Geometry check sheet. Reference: the model listing, model coordinates, mm. Face numbers are marked on the shaded views. A direction names the side the tool comes from. Round coordinates to 2 decimals unless told otherwise and drop trailing zeros. Write each loop counter-clockwise with the first axis right and the second up, starting at its lowest first coordinate (ties: lowest second). Pieces come first, ordered by that corner, then holes.
Item 1: Depth check by flat-ended pin: P1, Ø4, axis at x = -7.5, z = -12.5, coming from the +Y side; P2, Ø2, axis at x = 9, y = -10, coming from the -Z side; P3, Ø2, axis at x = -3, y = -20, coming from the +Z side. Enter the tip coordinate at first touch or a pass-through.
Item 2: Cross-section at B-B (y = -6). Enter the section's corners in (x, z), then the cut area to 3 significant figures.
Item 3: Cross-section at C-C (z = 9). Enter the section's corners in (x, y), then the cut area to 3 significant figures.
Item 4: Access from +Z, -Z, +X, -X, +Y, -Y to the whole of each face (thin tool, end or side, straight path). Record for the marked faces 1 and 2.
Item 5: Cross-section at D-D (x = -12.5). Enter the section's corners in (y, z).
Item 6: Scan lines: probe 1 along Y at (x, z) = (0.5, -20); probe 2 along Z at (x, y) = (0, 4); probe 3 along Z at (x, y) = (0.5, -20.5). Record each from-to range of solid material in increasing order.
Item 7: Cross-section at A-A (x = 0). Enter the section's corners in (y, z).
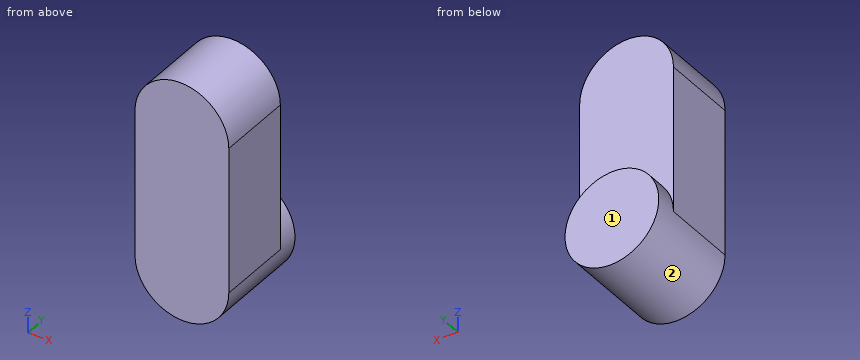
from build123d import *

# Parameters (mm, degrees)
F1_DEPTH = 7.24
F2_DEPTH = 25.4


with BuildPart() as f1:
    # F0 (on Front) → F1 (new body)
    with BuildSketch(Plane.XZ):
        with BuildLine():
            ThreePointArc((-16, -49.9569810927), (0, -65.9569810927), (16, -49.9569810927))
            ThreePointArc((16, -49.9569810927), (0, -33.9569810927), (-16, -49.9569810927))
        make_face()
    extrude(amount=-F1_DEPTH)

    # F0 (on Front) → F2 (join)
    with BuildSketch(Plane.XZ):
        with BuildLine():
            ThreePointArc((-16, 0), (0, -16), (16, 0))
            ThreePointArc((16, 0), (0, 16), (-16, 0))
        make_face()
        with BuildLine():
            Line((16, -49.9569810927), (16, 0))
            ThreePointArc((16, 0), (0, -16), (-16, 0))
            Line((-16, 0), (-16, -49.9569810927))
            ThreePointArc((-16, -49.9569810927), (0, -33.9569810927), (16, -49.9569810927))
        make_face()
        with BuildLine():
            ThreePointArc((-16, -49.9569810927), (0, -65.9569810927), (16, -49.9569810927))
            ThreePointArc((16, -49.9569810927), (0, -33.9569810927), (-16, -49.9569810927))
        make_face()
    extrude(amount=F2_DEPTH)


solid = f1.part
Resolved:
1. P1: stops at y = 0
1. P2: stops at z = -63.81
1. P3: stops at z = 15.87
2. outline: (-16, -49.96) arc R16 ccw to (16, -49.96) - (16, 0) arc R16 ccw to (-16, 0) - close
2. area: 2,400 mm2
3. outline: (-13.23, -25.4) - (13.23, -25.4) - (13.23, 0) - (-13.23, 0) - close
3. area: 672 mm2
4. face 1: +Z, -Z, +X, -X, +Y
4. face 2: +Y
5. outline: (-25.4, -59.94) - (7.24, -59.94) - (7.24, -39.97) - (0, -39.97) - (0, 9.99) - (-25.4, 9.99) - close
6. probe 1: y = -25.4 to 0
6. probe 2: z = -65.96 to -33.96
6. probe 3: z = -65.95 to 15.99
7. outline: (-25.4, -65.96) - (7.24, -65.96) - (7.24, -33.96) - (0, -33.96) - (0, 16) - (-25.4, 16) - close
